Geometry check sheet. Reference: the model listing, model coordinates, mm. Face numbers are marked on the shaded views. Coordinates: 2 decimals unless noted, no trailing zeros. Loops run counter-clockwise (first coordinate to the right, second up) from the corner with the lowest first, then second, coordinate; pieces in that order, holes last. Notation, with made-up numbers: (40.25, 89) -> (86.25, 89) arc R28 ccw to (86.25, 115) -> close; hole circle Ø4 at (23.25, 39.25). An arc over 180 degrees is marked (long way). Answer as a JSON object with one key per item and string values.
from build123d import *

# Parameters (mm, degrees)
F1_W      = 68
F1_H      = 129
F1_W_2    = 55
F1_H_2    = 100
F2_DEPTH  = 5
F3_R      = 3
F4_R      = 3
F5_W      = 55
F5_H      = 100
F6_DEPTH  = 3
F0_R      = 4.3933448382
F7_DEPTH  = 6
F8_W      = 4.1563683189
F8_H      = 5.0799995661
F9_DEPTH  = 6
F10_W     = 7.3890909553
F10_H     = 5.5418238044
F11_DEPTH = 6
F12_R     = 1.7585544961
F13_DEPTH = 6
F24_R     = 1.3854540884
F25_DEPTH = 6


# Not quite as in the source:
# - the program builds the solid bodies; features that only make, move or delete a surface that nothing else refers to are left out


with BuildPart() as f2:
    # F1 (on Top) → F2 (new body)
    with BuildSketch(Plane.XY):
        Rectangle(F1_W, F1_H)
        Rectangle(F1_W_2, F1_H_2, mode=Mode.SUBTRACT)
    extrude(amount=F2_DEPTH)

    # F3
    f3_edges = [f2.edges().sort_by_distance(p)[0] for p in [
        (-34, 64.5, 2.5),
        (34, 64.5, 2.5),
        (34, -64.5, 2.5),
        (-34, -64.5, 2.5),
    ]]
    fillet(f3_edges, radius=F3_R)

    # F4
    f4_edges = [f2.edges().sort_by_distance(p)[0] for p in [
        (-27.5, 50, 2.5),
        (27.5, 50, 2.5),
        (-27.5, -50, 2.5),
        (27.5, -50, 2.5),
    ]]
    fillet(f4_edges, radius=F4_R)

    # F5 (on Top) → F6 (join)
    with BuildSketch(Plane.XY):
        Rectangle(F5_W, F5_H)
    extrude(amount=F6_DEPTH)

    # F0 (on Top) → F7 (join)
    with BuildSketch(Plane.XY):
        with Locations((0, -58.5363544524)):
            Circle(F0_R)
    extrude(amount=F7_DEPTH)

    # F8 (on Top) → F9 (join)
    with BuildSketch(Plane.XY):
        with Locations((1.8472720403, 56.6872768104)):
            Rectangle(F8_W, F8_H)
    extrude(amount=F9_DEPTH)

    # F10 (on Top) → F11 (join)
    with BuildSketch(Plane.XY):
        with Locations((-6.4654545859, 57.1491010487)):
            Rectangle(F10_W, F10_H)
    extrude(amount=F11_DEPTH)

    # F12 (on Top) → F13 (join)
    with BuildSketch(Plane.XY):
        with Locations((26.3236332685, 57.8418262303)):
            Circle(F12_R)
    extrude(amount=F13_DEPTH)

    # F24 (on Top) → F25 (join)
    with BuildSketch(Plane.XY):
        with Locations((-30.4799992591, -60.15272066)):
            Circle(F24_R)
    extrude(amount=F25_DEPTH)


solid = f2.part
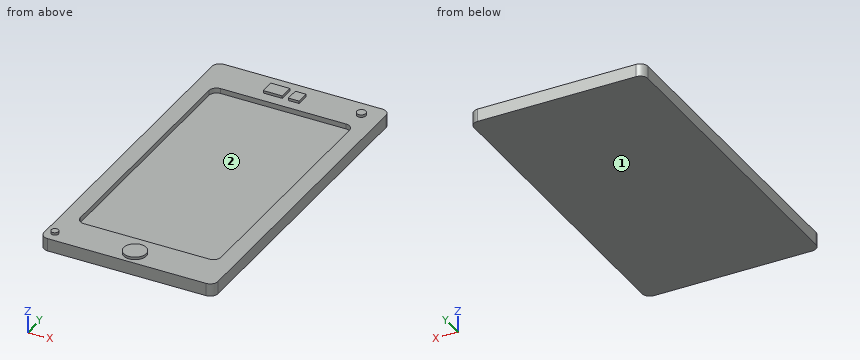
1. Mould release check, pull along X, two halves, no side actions. Record for the marked faces 1 and 2: released by +X, released by -X, zero draft, split by the parting line, or undercut.
Evaluation:
{"face 1": "zero draft", "face 2": "undercut"}
2. Section check A-A, the plane y = -30. Record the boundary of the cut face in (x, z), then the cut area to 3 significant figures.
Evaluation:
{"outline": "(-34, 0) -> (34, 0) -> (34, 5) -> (27.5, 5) -> (27.5, 3) -> (-27.5, 3) -> (-27.5, 5) -> (-34, 5) -> close", "area": "230 mm^2"}
3. Thickness scan on probe 1 along X at (y, z) = (18, 3.25); probe 2 along Y at (x, z) = (-21, 4.7); probe 3 along Z at (x, y) = (-4, 51.5). Record the ranges inside material, lowest first. Write a range as from..to.
Evaluation:
{"probe 1": "x = -34..-27.5, 27.5..34", "probe 2": "y = -64.5..-50, 50..64.5", "probe 3": "z = 0..5"}
4. Depth check by flat-ended pin: P1, Ø20.5, axis at x = -12, y = 2, coming from the +Z side; P2, Ø0.8, axis at y = 56.5, z = 5.5, coming from the +X side; P3, Ø0.8, axis at x = 2.5, z = 5.5, coming from the -Y side. Enter the tip coordinate at first touch or a pass-through.
Evaluation:
{"P1": "stops at z = 3", "P2": "stops at x = 27.81", "P3": "stops at y = -62.4"}
5. Section check B-B, the plane x = 9. Record the boundary of the cut face in (y, z), then the cut area to 3 significant figures.
Evaluation:
{"outline": "(-64.5, 0) -> (64.5, 0) -> (64.5, 5) -> (50, 5) -> (50, 3) -> (-50, 3) -> (-50, 5) -> (-64.5, 5) -> close", "area": "445 mm^2"}
